from build123d import *

# Parameters (mm, degrees)
SKETCH1_R           = 14
BOSS_EXTRUDE1_DEPTH = 15
CHAMFER1_SIZE       = 2.38
SKETCH3_R           = 2.5
BOSS_EXTRUDE2_DEPTH = 13.97
SKETCH5_R           = 1.75
BOSS_EXTRUDE4_DEPTH = 10


with BuildPart() as part:
    # Sketch1 → Boss-Extrude1 (new body)
    with BuildSketch(Plane.XY):
        Circle(SKETCH1_R)
    extrude(amount=BOSS_EXTRUDE1_DEPTH)

    # Chamfer1
    chamfer1_edges = [part.edges().sort_by_distance(p)[0] for p in [
        (-14, 0, 0),
        (-14, 0, 15),
    ]]
    chamfer(chamfer1_edges, length=CHAMFER1_SIZE)

    # Sketch3 → Boss-Extrude2 (add)
    with BuildSketch(Plane.XY.offset(15)):
        Circle(SKETCH3_R)
    extrude(amount=BOSS_EXTRUDE2_DEPTH)

    # Sketch5 → Boss-Extrude4 (add)
    with BuildSketch(Plane(origin=(0, 0, 0), x_dir=(-1, 0, 0), z_dir=(0, 0, -1))):
        with Locations((-9.5, 0)):
            Circle(SKETCH5_R)
        with Locations((9.5, 0)):
            Circle(SKETCH5_R)
    extrude(amount=BOSS_EXTRUDE4_DEPTH)


solid = part.part
Input: part model. Units: mm. Frame: model coordinates. A direction names the side the tool comes from. Give positions to 0.01 mm unless a question says otherwise; leave off trailing zeros. Write each loop counter-clockwise with the first axis right and the second up, starting at its lowest first coordinate (ties: lowest second). Pieces come first, ordered by that corner, then holes.
Q1. Pull-direction query (X, two-part tool) for faces 4 (the face through (-2.54, -11.46, 14.88)), 5 (the face through (0, 0, 28.97)), 6 (the face through (-11.169, 0.526, -4.93)); classes: pulls with the +X half, pulls with the -X half, needs draft (parallel to the pull), parting line crosses it, or undercut.
Q2. Section B-B, the plane z = -4.5. Output: boundary loops of the cut face in (x, y), plus the area to 3 significant figures.
Q3. Material intervals for probe 1 along Z at (x, y) = (1.5, -8.75); probe 2 along Z at (x, y) = (-1.5, 0.75); probe 3 along Y at (x, z) = (0, 22), sorted ascending.
Q4. Set-up query: faces 1 (the face through (7.831, 0.526, -4.93)), 2 (the face through (-0.54, -2.44, 21.89)), 3 (the face through (10, 0, -10)). Return all of +Z, -Z, +X, -X, +Y, -Y with unobstructed straight access to the full face (end or side cutting, diameter ignored); none if empty.
Q5. Section A-A, the plane x = 0. Output: boundary loops of the cut face in (y, z), plus the area to 3 significant figures.
Q6. Section D-D, the plane z = 0.5. Output: boundary loops of the cut face in (x, y), plus the area to 3 significant figures.
Q7. First-contact query: P1, Ø3, axis at x = 5, z = 11, coming from the +Y side; P2, Ø1, axis at y = 1.5, z = 19, coming from the +X side; P3, Ø5, axis at y = -5.5, z = 15.5, coming from the -X side. Flat tips, straight axial feed; report the tip coordinate or a pass-through.
Q8. Section C-C, the plane y = 0. Output: boundary loops of the cut face in (x, z).
Filled in:
1. face 4: parting line crosses it
1. face 5: needs draft
1. face 6: undercut
2. outline: circle Ø3.5 at (-9.5, 0); circle Ø3.5 at (9.5, 0)
2. area: 19.2 mm2
3. probe 1: z = 0 to 15
3. probe 2: z = 0 to 28.97
3. probe 3: y = -2.5 to 2.5
4. face 1: -Z
4. face 2: +Z
4. face 3: -Z, +X, -X, +Y, -Y
5. outline: (-14, 2.38) - (-11.62, 0) - (11.62, 0) - (14, 2.38) - (14, 12.62) - (11.62, 15) - (2.5, 15) - (2.5, 28.97) - (-2.5, 28.97) - (-2.5, 15) - (-11.62, 15) - (-14, 12.62) - close
5. area: 479 mm2
6. outline: circle Ø24.24 at (0, 0)
6. area: 461 mm2
7. P1: stops at y = 13.56
7. P2: stops at x = 2.29
7. P3: stops at x = -12.64
8. outline: (-14, 2.38) - (-11.62, 0) - (-11.25, 0) - (-11.25, -10) - (-7.75, -10) - (-7.75, 0) - (7.75, 0) - (7.75, -10) - (11.25, -10) - (11.25, 0) - (11.62, 0) - (14, 2.38) - (14, 12.62) - (11.62, 15) - (2.5, 15) - (2.5, 28.97) - (-2.5, 28.97) - (-2.5, 15) - (-11.62, 15) - (-14, 12.62) - close
